Design review of the part built by this model. Coordinates are the model's own, in mm. Coordinates: 2 decimals unless noted, no trailing zeros. Loops run counter-clockwise (first coordinate to the right, second up) from the corner with the lowest first, then second, coordinate; pieces in that order, holes last. Notation, with made-up numbers: M 58.5,62 L 84.5,62 A20 ccw 84.5,67 Z; hole C 9,83 d4. An arc over 180 degrees is marked long. Put each result on its own line as item: value. Start each with the question number.
(1) The part is to be moulded in two halves that separate along Z. For faces 1 (the flat face through (-3.893, -1.503, 10.504)), 2 (the cylindrical face through (55.145, -1.503, -18.247)), 3 (the flat face through (17.8, -1.5, 18)), 4 (the flat face through (10, -3.048, 40)), say which applies: +Z half, -Z half, draft (parallel to the pull), parting line (faces both ways), or undercut.
(2) Take a section at C-C, the plane z = -9. Give the boundary of the cut face in (x, y).
(3) Take a section at B-B, the plane y = -2.55. Count the separate pieces of the cut face and the enclosed holes in it, then the cut area to 3 significant figures.
(4) Take a section at D-D, the plane x = -4. Give the boundary of the cut face in (y, z), then the cut area to 3 significant figures.
(5) Take a section at A-A, the plane x = 20. Give the boundary of the cut face in (y, z).
(6) For probe 1 along Z at (x, y) = (6, -1.8); probe 2 along X at (y, z) = (-1.35, -20); probe 3 along X at (y, z) = (-2.25, -17.5), list the stretches that pass through material, from the lowest coordinate up. Write a range as [from, to].
```python
from build123d import *

# Parameters (mm, degrees)
F1_DEPTH = 3.048


with BuildPart() as f1:
    # F0 (on Front) → F1 (new body)
    with BuildSketch(Plane.XZ):
        with BuildLine():
            ThreePointArc((7.5227019244, -10.4490181237), (1.5890806412, -13.1143226875), (-0.3596819621, -19.3202903209))
            ThreePointArc((-0.3596819621, -19.3202903209), (2.2826274956, -24.3485250199), (7.6084325525, -26.3235551344))
            ThreePointArc((7.6084325525, -26.3235551344), (13.16559095, -23.9687855568), (15.4602019244, -18.3865181237))
            Line((15.4602019244, -18.3865181237), (10.6977019244, -18.3865181237))
            ThreePointArc((10.6977019244, -18.3865181237), (5.2776378942, -20.631582154), (7.5227019244, -15.2115181237))
            Line((7.5227019244, -15.2115181237), (7.5227019244, -10.4490181237))
        make_face()
        with BuildLine():
            Line((14.2200019541, -1.0290787363), (21.4755552782, 37.5415925289))
            ThreePointArc((21.4755552782, 37.5415925289), (15.6409493218, 31.4712795543), (7.5227019244, 29.2384818763))
            Line((7.5227019244, 29.2384818763), (7.5227019244, -10.4490181237))
            ThreePointArc((7.5227019244, -10.4490181237), (13.1353620001, -12.7738580481), (15.4602019244, -18.3865181237))
            Line((15.4602019244, -18.3865181237), (44.0352019244, -18.3865181237))
            ThreePointArc((44.0352019244, -18.3865181237), (46.3600418488, -12.7738580481), (51.9727019244, -10.4490181237))
            Line((51.9727019244, -10.4490181237), (22.0331668809, -10.4490181237))
            ThreePointArc((22.0331668809, -10.4490181237), (15.9139184745, -7.5742963259), (14.2200019541, -1.0290787363))
        make_face()
        with BuildLine():
            ThreePointArc((-1.9275910398, 97.1041068763), (0.3789519244, 89.6132865668), (7.5227019244, 86.3884818763))
            ThreePointArc((7.5227019244, 86.3884818763), (14.2578940152, 89.1782897855), (17.0477019244, 95.9134818763))
            ThreePointArc((17.0477019244, 95.9134818763), (17.0290068187, 96.5099651182), (16.9729948886, 97.1041068763))
            ThreePointArc((16.9729948886, 97.1041068763), (7.5227019244, 105.4384818763), (-1.9275910398, 97.1041068763))
        make_face()
        with BuildLine():
            ThreePointArc((10.6977019244, 95.9134818763), (9.7677659547, 93.668417846), (7.5227019244, 92.7384818763))
            ThreePointArc((7.5227019244, 92.7384818763), (5.2776378942, 98.1585459065), (10.6977019244, 95.9134818763))
        make_face(mode=Mode.SUBTRACT)
        with BuildLine():
            ThreePointArc((59.9102019244, -18.3865181237), (57.5853620001, -12.7738580481), (51.9727019244, -10.4490181237))
            ThreePointArc((51.9727019244, -10.4490181237), (46.3600418488, -12.7738580481), (44.0352019244, -18.3865181237))
            ThreePointArc((44.0352019244, -18.3865181237), (46.3600125617, -23.9991489122), (51.9726190879, -26.3240181233))
            ThreePointArc((51.9726190879, -26.3240181233), (57.5853327129, -23.9992074864), (59.9102019244, -18.3865181237))
        make_face()
        with BuildLine():
            ThreePointArc((55.1477019244, -18.3865181237), (51.9727019244, -21.5615181237), (48.7977019244, -18.3865181237))
            ThreePointArc((48.7977019244, -18.3865181237), (51.9727019244, -15.2115181237), (55.1477019244, -18.3865181237))
        make_face(mode=Mode.SUBTRACT)
        with BuildLine():
            ThreePointArc((23.2731901981, 47.0978568763), (18.0230274402, 57.0197318763), (7.5227019244, 60.9884818763))
            Line((7.5227019244, 60.9884818763), (7.5227019244, 48.2884818763))
            ThreePointArc((7.5227019244, 48.2884818763), (9.7677659547, 47.3585459065), (10.6977019244, 45.1134818763))
            ThreePointArc((10.6977019244, 45.1134818763), (9.7677659547, 42.868417846), (7.5227019244, 41.9384818763))
            Line((7.5227019244, 41.9384818763), (7.5227019244, 29.2384818763))
            ThreePointArc((7.5227019244, 29.2384818763), (15.6409493218, 31.4712795543), (21.4755552782, 37.5415925289))
            Line((21.4755552782, 37.5415925289), (23.2731901981, 47.0978568763))
        make_face()
        with BuildLine():
            ThreePointArc((23.3977019244, 45.1134818763), (23.3665434148, 46.1076206129), (23.2731901981, 47.0978568763))
            Line((23.2731901981, 47.0978568763), (21.4755552782, 37.5415925289))
            ThreePointArc((21.4755552782, 37.5415925289), (22.9096634827, 41.2074558901), (23.3977019244, 45.1134818763))
        make_face()
        with BuildLine():
            ThreePointArc((17.0477019244, 95.9134818763), (14.2578940152, 89.1782897855), (7.5227019244, 86.3884818763))
            Line((7.5227019244, 86.3884818763), (7.5227019244, 60.9884818763))
            ThreePointArc((7.5227019244, 60.9884818763), (18.0230274402, 57.0197318763), (23.2731901981, 47.0978568763))
            Line((23.2731901981, 47.0978568763), (16.9729948886, 97.1041068763))
            ThreePointArc((16.9729948886, 97.1041068763), (17.0290068187, 96.5099651182), (17.0477019244, 95.9134818763))
        make_face()
        with BuildLine():
            ThreePointArc((15.4602019244, -18.3865181237), (13.1353620001, -12.7738580481), (7.5227019244, -10.4490181237))
            Line((7.5227019244, -10.4490181237), (7.5227019244, -15.2115181237))
            ThreePointArc((7.5227019244, -15.2115181237), (9.7677659547, -16.1414540935), (10.6977019244, -18.3865181237))
            Line((10.6977019244, -18.3865181237), (15.4602019244, -18.3865181237))
        make_face()
        with BuildLine():
            ThreePointArc((15.4602019244, -18.3865181237), (13.16559095, -23.9687855568), (7.6084325525, -26.3235551344))
            Line((7.6084325525, -26.3235551344), (51.9726190879, -26.3240181233))
            ThreePointArc((51.9726190879, -26.3240181233), (46.3600125617, -23.9991489122), (44.0352019244, -18.3865181237))
            Line((44.0352019244, -18.3865181237), (15.4602019244, -18.3865181237))
        make_face()
        with BuildLine():
            Line((7.5227019244, 48.2884818763), (7.5227019244, 60.9884818763))
            ThreePointArc((7.5227019244, 60.9884818763), (-2.9776235914, 57.0197318763), (-8.2277863493, 47.0978568763))
            Line((-8.2277863493, 47.0978568763), (-7.3281904539, 39.5039702604))
            ThreePointArc((-7.3281904539, 39.5039702604), (-1.5040535308, 32.0546415391), (7.5227019244, 29.2384818763))
            Line((7.5227019244, 29.2384818763), (7.5227019244, 41.9384818763))
            ThreePointArc((7.5227019244, 41.9384818763), (4.3477019244, 45.1134818763), (7.5227019244, 48.2884818763))
        make_face()
        with BuildLine():
            Line((7.5227019244, 60.9884818763), (7.5227019244, 86.3884818763))
            ThreePointArc((7.5227019244, 86.3884818763), (0.3789519244, 89.6132865668), (-1.9275910398, 97.1041068763))
            Line((-1.9275910398, 97.1041068763), (-8.2277863493, 47.0978568763))
            ThreePointArc((-8.2277863493, 47.0978568763), (-2.9776235914, 57.0197318763), (7.5227019244, 60.9884818763))
        make_face()
        with BuildLine():
            ThreePointArc((7.5227019244, 29.2384818763), (-1.5040535308, 32.0546415391), (-7.3281904539, 39.5039702604))
            Line((-7.3281904539, 39.5039702604), (-0.3596819621, -19.3202903209))
            ThreePointArc((-0.3596819621, -19.3202903209), (1.5890806412, -13.1143226875), (7.5227019244, -10.4490181237))
            Line((7.5227019244, -10.4490181237), (7.5227019244, 29.2384818763))
        make_face()
        with BuildLine():
            Line((-7.3281904539, 39.5039702604), (-8.2277863493, 47.0978568763))
            ThreePointArc((-8.2277863493, 47.0978568763), (-8.2420658485, 43.245937482), (-7.3281904539, 39.5039702604))
        make_face()
    extrude(amount=F1_DEPTH)


solid = f1.part
```
Computed values:
1. face 1: -Z half
1. face 2: undercut
1. face 3: undercut
1. face 4: draft
2. outline: M -1.58,-3.05 L 17.46,-3.05 L 17.46,0 L -1.58,0 Z
3. separate pieces: 1
3. enclosed holes: 4
3. area: 3,510 mm^2
4. outline: M -3.05,11.41 L 0,11.41 L 0,80.65 L -3.05,80.65 Z
4. area: 211 mm^2
5. outline: M -3.05,-26.32 L 0,-26.32 L 0,-10.18 L -3.05,-10.18 Z; M -3.05,29.7 L 0,29.7 L 0,73.08 L -3.05,73.08 Z
6. probe 1: z = [-26.18, -21.17], [-15.6, 42.33], [47.9, 93.13], [98.7, 105.32]
6. probe 2: x = [-0.25, 4.79], [10.26, 49.24], [54.71, 59.74]
6. probe 3: x = [-0.58, 4.47], [10.57, 48.92], [55.02, 59.86]
